Work out the finished part from the listing and answer in its coordinate system (mm). A direction names the side the tool comes from. Round coordinates to 2 decimals unless told otherwise and drop trailing zeros. Order: outer loops, then holes, each group sorted by start corner. A loop starts at its lowest first (then second) coordinate and runs counter-clockwise, first axis right, second up.
from build123d import *

# Parameters (mm, degrees)
SKETCH1_R           = 12.5
SKETCH1_R_2         = 9
BOSS_EXTRUDE1_DEPTH = 80
SKETCH2_R           = 3.5
BOSS_EXTRUDE2_DEPTH = 5


with BuildPart() as part:
    # Sketch1 → Boss-Extrude1 (new body)
    with BuildSketch(Plane.XY):
        Circle(SKETCH1_R)
        Circle(SKETCH1_R_2, mode=Mode.SUBTRACT)
    extrude(amount=BOSS_EXTRUDE1_DEPTH)

    # Sketch2 → Boss-Extrude2 (add, symmetric)
    with BuildSketch(Plane(origin=(0, 0, 0), x_dir=(1, 0, 0), z_dir=(0, 1, 0))):
        with BuildLine():
            Line((-12.5, 0), (12.5, 0))
            Line((12.5, 0), (12.5, 25))
            ThreePointArc((12.5, 25), (0, 37.5), (-12.5, 25))
            Line((-12.5, 25), (-12.5, 0))
        make_face()
        with Locations((0, 25)):
            Circle(SKETCH2_R, mode=Mode.SUBTRACT)
    extrude(amount=BOSS_EXTRUDE2_DEPTH, both=True)


solid = part.part
Item 1: Find section A-A (x = 0). Write down the section's boundary in (y, z), plus the area to 3 significant figures.
Item 2: Given pin 1 (12 mm diameter, centred on x = -2, z = -21.5, fed in from +Y); pin 2 (2 mm diameter, centred on x = 1.5, y = -8.5, fed in from +Z); pin 3 (5 mm diameter, centred on x = -2.5, y = 0.5, fed in from +Z); pin 4 (4 mm diameter, centred on x = 4, z = 2.5, fed in from +Y), each flat-ended and moving along its own axis, determine where each tip first touches the part or whether it passes through.
Item 3: Find section B-B (y = -6.75). Write down the section's boundary in (x, z).
Item 4: Find the intervals of material crossed by line 1 along Z through (x, y) = (0, 0.75); line 2 along Y through (x, z) = (0, 28.5); line 3 along X through (y, z) = (-1.5, -25), in increasing order.
Item 5: For a pull along X with two mould halves and no side action, classify faces 5 (the face through (-0.46, -0.07, -28.47)), 6 (the face through (0.275, 0.07, -37.497)), 7 (the face through (0, 10, 0)) as released by +X, released by -X, zero draft, split by the parting line, or undercut.
Item 6: Find section D-D (y = 1). Write down the section's boundary in (x, z).
Item 7: Find section C-C (z = 36). Write down the section's boundary in (x, y), plus the area to 3 significant figures.
Item 8: A tool of negligible diameter and unlimited length cuts with its end or side. For faces 1 (the face through (12.5, 0, -12)), 2 (the face through (0, 5, -19)), 3 (the face through (0, -10, 0)), 4 (the face through (0, 0, 0)), from which of +Z, -Z, +X, -X, +Y, -Y can it reach the whole face along a straight path? Write none if from no direction.
Model answer:
1. outline: (-12.5, 0) - (-9, 0) - (-9, 80) - (-12.5, 80) - close; (-5, -37.5) - (5, -37.5) - (5, -28.5) - (-5, -28.5) - close; (-5, -21.5) - (5, -21.5) - (5, 0) - (-5, 0) - close; (9, 0) - (12.5, 0) - (12.5, 80) - (9, 80) - close
1. area: 865 mm2
2. pin 1: stops at y = 5
2. pin 2: stops at z = 80
2. pin 3: stops at z = 0
2. pin 4: stops at y = 12.34
3. outline: (-10.52, 0) - (-5.95, 0) - (-5.95, 80) - (-10.52, 80) - close; (5.95, 0) - (10.52, 0) - (10.52, 80) - (5.95, 80) - close
4. line 1: z = -37.5 to -28.5, -21.5 to 0
4. line 2: y = -12.5 to -9, 9 to 12.5
4. line 3: x = -12.5 to -3.5, 3.5 to 12.5
5. face 5: undercut
5. face 6: split by the parting line
5. face 7: zero draft
6. outline: (-12.5, -25) arc R12.5 ccw to (12.5, -25) - (12.5, 0) - (12.46, 0) - (12.46, 80) - (8.94, 80) - (8.94, 0) - (-8.94, 0) - (-8.94, 80) - (-12.46, 80) - (-12.46, 0) - (-12.5, 0) - close; hole circle Ø7 at (0, -25)
7. outline: circle Ø25 at (0, 0); hole circle Ø18 at (0, 0)
7. area: 236 mm2
8. face 1: +Z, -Z, +X, +Y, -Y
8. face 2: -Z, +X, -X, +Y
8. face 3: -Z, +X, -X, -Y
8. face 4: +Z
